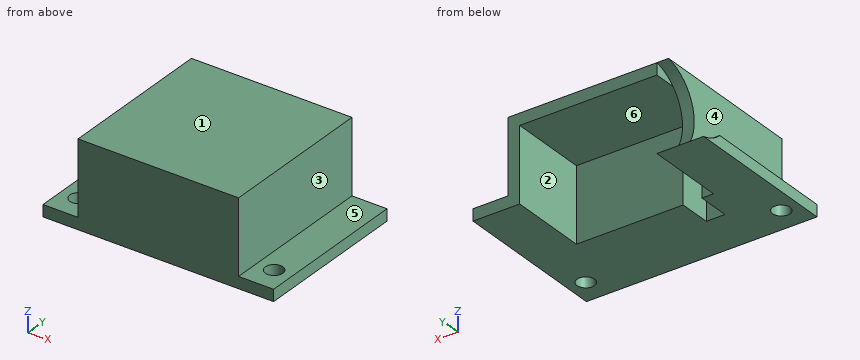
```python
from build123d import *

# Parameters (mm, degrees)
BOSS_EXTRUDE1_DEPTH = 12.7
SKETCH2_W           = 39.5
SKETCH2_H           = 27
BOSS_EXTRUDE2_DEPTH = 2
SKETCH3_W           = 6
SKETCH3_H           = 12.7
CUT_EXTRUDE1_DEPTH  = 38.396997736
CUT_EXTRUDE2_START  = -2
CUT_EXTRUDE2_DEPTH  = 12
SKETCH5_R           = 1.5
CUT_EXTRUDE3_DEPTH  = 33.837341068


with BuildPart() as part:
    # Sketch1 → Boss-Extrude1 (new body)
    with BuildSketch(Plane.XY):
        Polygon((-10.205741627, 6.782296651), (-10.205741627, -6.717703349), (-8.205741627, -6.717703349), (-8.205741627, -12.217703349), (-5.005741627, -12.217703349), (-5.005741627, -6.717703349), (13.294258373, -6.717703349), (13.294258373, 6.782296651), (21.294258373, 6.782296651), (21.294258373, -20.217703349), (-18.205741627, -20.217703349), (-18.205741627, 6.782296651), align=None)
    extrude(amount=BOSS_EXTRUDE1_DEPTH)

    # Sketch2 → Boss-Extrude2 (add)
    with BuildSketch(Plane.XY.offset(12.7)):
        with Locations((1.544258373, -6.717703349)):
            Rectangle(SKETCH2_W, SKETCH2_H)
    extrude(amount=BOSS_EXTRUDE2_DEPTH)

    # Sketch3 → Cut-Extrude1 (cut, through all)
    with BuildSketch(Plane(origin=(0, 6.782296651, 0), x_dir=(1, 0, 0), z_dir=(0, 1, 0))):
        with Locations((-15.205741627, -8.35)):
            Rectangle(SKETCH3_W, SKETCH3_H)
        with Locations((18.294258373, -8.35)):
            Rectangle(SKETCH3_W, SKETCH3_H)
    extrude(amount=-CUT_EXTRUDE1_DEPTH, mode=Mode.SUBTRACT)

    # Sketch4 → Cut-Extrude2 (cut)
    with BuildSketch(Plane.ZY.offset(12.205741627).offset(CUT_EXTRUDE2_START)):
        with BuildLine():
            Line((0, 6.782296651), (14.7, 6.782296651))
            ThreePointArc((14.7, 6.782296651), (7.35, 0.679443812), (0, 6.782296651))
        make_face()
    extrude(amount=CUT_EXTRUDE2_DEPTH, mode=Mode.SUBTRACT)

    # Sketch5 → Cut-Extrude3 (cut, through all)
    with BuildSketch(Plane(origin=(0, 0, 0), x_dir=(-1, 0, 0), z_dir=(0, 0, -1))):
        with Locations((-18.294258373, -15.917381118)):
            Circle(SKETCH5_R)
        with Locations((15.205741627, -15.917381118)):
            Circle(SKETCH5_R)
    extrude(amount=-CUT_EXTRUDE3_DEPTH, mode=Mode.SUBTRACT)


solid = part.part
```
Source: CAD feature listing. Evaluate the final solid. Frame: model axes, mm. Face numbers are marked on the shaded views. A direction names the side the tool comes from. Give positions to 0.01 mm unless a question says otherwise; leave off trailing zeros. Loops run counter-clockwise (first coordinate to the right, second up) from the corner with the lowest first, then second, coordinate; pieces in that order, holes last. Notation, with made-up numbers: M -32.5,-23 L -21.5,-23 A26 cw -21.5,12 Z; hole C 7,-6.5 d7. An arc over 180 degrees is marked long. Put each result on its own line as item: value.
Q1. Section C-C (y = -16.75). Return the cut outline in (x, z), and give its area (3 significant figures).
Response values:
outline: M -18.21,0 L -16.45,0 L -16.45,2 L -18.21,2 Z; M -13.96,0 L 17.05,0 L 17.05,2 L 15.29,2 L 15.29,14.7 L -12.21,14.7 L -12.21,2 L -13.96,2 Z; M 19.54,0 L 21.29,0 L 21.29,2 L 19.54,2 Z
area: 418 mm²
Q2. Section D-D (z = 8.25). Return the cut outline in (x, y), and give its area (3 significant figures).
Response values:
outline: M -12.21,-20.22 L 15.29,-20.22 L 15.29,6.78 L 13.29,6.78 L 13.29,-6.72 L -5.01,-6.72 L -5.01,-12.22 L -8.21,-12.22 L -8.21,-6.72 L -10.21,-6.72 L -10.21,0.73 L -12.21,0.73 Z
area: 396 mm²
Q3. Pin query (flat end, axial travel): P1, Ø2.5, axis at x = -6.5, z = 4, coming from the +Y side; P2, Ø15, axis at x = 2, y = 1, coming from the -Z side; P3, Ø1, axis at x = 5, y = -14.5, coming from the -Z side; P4, Ø1.5, axis at y = -14.5, z = 12.5, coming from the +X side. Return the tip coordinate at first contact, or that it passes through.
Response values:
P1: stops at y = -12.22
P2: stops at z = 12.7
P3: stops at z = 0
P4: stops at x = 15.29
Q4. Line query: probe 1 along X at (y, z) = (0, 8); probe 2 along X at (y, z) = (-8, 9.25); probe 3 along Z at (x, y) = (17, -10.25). Output: solid intervals per line, ascending. Write a range as [from, to].
Response values:
probe 1: x = [-12.21, -10.21], [13.29, 15.29]
probe 2: x = [-12.21, -8.21], [-5.01, 15.29]
probe 3: z = [0, 2]
Q5. Section A-A (y = 3.5). Return the cut outline in (x, z).
Response values:
outline: M -18.21,0 L -10.21,0 L -10.21,1.5 L -18.21,1.5 Z; M -12.21,13.2 L -10.21,13.2 L -10.21,12.7 L 13.29,12.7 L 13.29,0 L 21.29,0 L 21.29,2 L 15.29,2 L 15.29,14.7 L -12.21,14.7 Z
Q6. Mould query, pull axis X, two halves, no side actions, for the marked faces 4, 5 and 6. Classes: released by +X, released by -X, zero draft, split by the parting line, or undercut.
Response values:
face 4: released by -X
face 5: zero draft
face 6: undercut
Q7. Section B-B (x = -14.5). Return the cut outline in (y, z).
Response values:
outline: M -20.22,0 L -17.24,0 L -17.24,2 L -20.22,2 Z; M -14.59,0 L 6.78,0 A7.48 cw 2.93,2 L -14.59,2 Z
Q8. Reachability of the marked faces 1, 2 and 3 from +Z, -Z, +X, -X, +Y, -Y: full face, straight path, thin tool, end or side. Return the list, or none.
Response values:
face 1: +Z, +X, -X, +Y, -Y
face 2: -Z, +Y
face 3: +Z, +X, +Y, -Y
